Geometry check sheet. Reference: drawing and pictorial views, mm from the part's lowest x, y, z. A direction names the side the tool comes from. Round coordinates to 2 decimals unless told otherwise and drop trailing zeros. Order: outer loops, then holes, each group sorted by start corner. A loop starts at its lowest first (then second) coordinate and runs counter-clockwise, first axis right, second up. Notation, with made-up numbers: M -32.5,12 L 1.5,12 A18 cw 1.5,18 Z; hole C 19,-37.75 d3. An arc over 180 degrees is marked long. Answer as a JSON object with one key per item and string values. Group by question number.
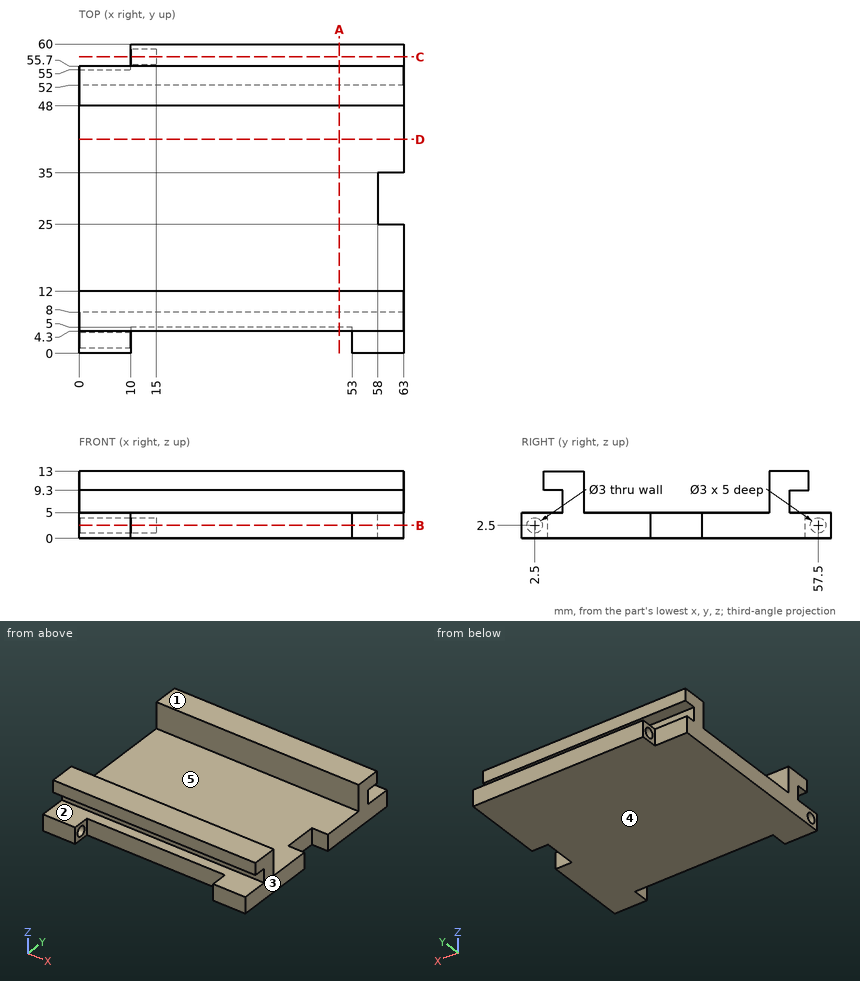
Q1. Cross-section at A-A, the plane x = 50.5. Record the cut outline in (y, z), then the cut area to 3 significant figures.
Q2. Cross-section at D-D, the plane y = 41.5. Record the cut outline in (x, z).
Q3. Gauge pin test, flat ends, axial feed: pin 1 Ø8 at (x, y) = (19.5, 15) entering from +Z; pin 2 Ø2.5 at (y, z) = (31, 2.5) entering from +X; pin 3 Ø1.3 at (x, z) = (27, 7) entering from -Y; pin 4 Ø2.5 at (y, z) = (57.5, 2.5) entering from -X. Record the tip position at first contact, or that the pin passes through.
Q4. Thickness scan on line 1 (Y direction, x = 25, z = 12); line 2 (Y direction, x = 12.5, z = 6.5); line 3 (X direction, y = 3, z = 4). Record the ranges inside material, lowest first. Write a range as from..to.
Q5. Cross-section at C-C, the plane y = 57.5. Record the cut outline in (x, z), then the cut area to 3 significant figures.
Q6. Release check for a two-part mould opening along Z. For the marked faces 1, 2 and 3 record: released by +Z, released by -Z, zero draft, split by the parting line, or undercut.
Q7. Cross-section at B-B, the plane z = 2.5. Record the cut outline in (x, y), then the cut area to 3 significant figures.
Q8. Tool access check on the marked faces 4 and 5. Record the directions out of +Z, -Z, +X, -X, +Y, -Y that give a thin tool (end or side, any length) a straight path to the whole face; none if there is none.
Conclusion:
{
 "1": {"outline": "M 4.3,9.3 L 8,9.3 L 8,5 L 5,5 L 5,0 L 60,0 L 60,5 L 52,5 L 52,9.3 L 55.7,9.3 L 55.7,13 L 48,13 L 48,5 L 12,5 L 12,13 L 4.3,13 Z", "area": "366 mm2"},
 "2": {"outline": "M 0,0 L 63,0 L 63,5 L 0,5 Z"},
 "3": {"pin 1": "z = 13", "pin 2": "x = 58", "pin 3": "y = 8", "pin 4": "x = 15"},
 "4": {"line 1": "4.3..12, 48..55.7", "line 2": "8..12, 48..52", "line 3": "0..10, 53..63"},
 "5": {"outline": "M 10,0 L 63,0 L 63,5 L 10,5 L 10,4 L 15,4 L 15,1 L 10,1 Z", "area": "250 mm2"},
 "6": {"face 1": "released by +Z", "face 2": "undercut", "face 3": "zero draft"},
 "7": {"outline": "M 0,0 L 10,0 L 10,1 L 0,1 Z; M 0,4 L 10,4 L 10,5 L 53,5 L 53,0 L 63,0 L 63,25 L 58,25 L 58,35 L 63,35 L 63,60 L 10,60 L 10,59 L 15,59 L 15,56 L 10,56 L 10,55 L 0,55 Z", "area": "3,420 mm2"},
 "8": {"face 4": "-Z, +X, -X, +Y, -Y", "face 5": "+Z, +X, -X"}
}
